CAD build for the part. Positions are in the model's coordinates, mm. A direction names the side the tool comes from. Round coordinates to 2 decimals unless told otherwise and drop trailing zeros. Order: outer loops, then holes, each group sorted by start corner. A loop starts at its lowest first (then second) coordinate and runs counter-clockwise, first axis right, second up. Notation, with made-up numbers: (79, 88.25) - (95, 88.25) arc R27 cw to (95, 119.25) - close; hole circle Ø11 at (-32, -28.5). An arc over 180 degrees is marked (long way). Use one line per item in the form item = value. Start each with the question number.
from build123d import *

# Parameters (mm, degrees)
F0_R     = 9.525
F1_DEPTH = 9.525
F2_DEPTH = 88.9
F3_DEPTH = 25.4


with BuildPart() as f1:
    # F0 (on Front) → F1 (new body)
    with BuildSketch(Plane.XZ):
        Polygon((-4.2214523455, 17.4378681917), (-17.2123630146, 5.0630491238), (-12.9909106691, -12.3748190679), (4.2214523455, -17.4378681917), (17.2123630146, -5.0630491238), (12.9909106691, 12.3748190679), align=None)
        Circle(F0_R, mode=Mode.SUBTRACT)
        Circle(F0_R)
    extrude(amount=F1_DEPTH)

    # F0 (on Front) → F2 (join)
    with BuildSketch(Plane.XZ):
        Circle(F0_R)
    extrude(amount=F2_DEPTH)

    # F3 (add): a face of the model
    f3_faces = [f1.faces().sort_by_distance(p)[0] for p in [
        (0, -88.9, 0),
    ]]
    extrude(f3_faces, amount=F3_DEPTH)


solid = f1.part
(1) Flat gauge pins, fed straight in: P1, Ø4, axis at x = -1, y = -55.5, coming from the -Z side (3 decimals); P2, Ø5, axis at y = -70, z = -9, coming from the -X side; P3, Ø2, axis at y = -33, z = -5, coming from the -X side. Where does each tip first touch, or does it go through?
(2) Slice it at B-B (y = -93.5). Give the cut face in (x, z) (3 decimals), and give its area (3 significant figures).
(3) Wall check: line 1 (Y direction, x = 9.5, z = 2.5) (3 decimals); line 2 (X direction, y = -65, z = -1); line 3 (Z direction, x = 4.5, y = -28). Give the ranges that are in metal, low to high. Write a range as [from, to].
(4) Which spindle directions (+Z, -Z, +X, -X, +Y, -Y) get a long thin tool onto all of the face, cutting with end or side? Do faces 1 (the flat face through (10.626, -4.696, -11.337)), 2 (the cylindrical face through (-7.559, -61.179, -5.796)). Say none if no direction does.
(5) Slice it at C-C (x = 2.5). Give the cut face in (y, z) (1 decimal).
(6) Slice it at A-A (z = 0). Give the cut face in (x, y) (3 decimals), and give its area (3 significant figures).
Results list:
q1.P1 = -9.525
q1.P2 = -6.96
q1.P3 = -8.64
q2.outline = circle Ø19.05 at (0, 0)
q2.area = 285 mm²
q3.line_1 = [-9.525, 0]
q3.line_2 = [-9.47, 9.47]
q3.line_3 = [-8.39, 8.39]
q4.face_1 = -Z, +X, +Y, -Y
q4.face_2 = -Y
q5.outline = (-114.3, -9.2) - (-9.5, -9.2) - (-9.5, -16.9) - (0, -16.9) - (0, 15.5) - (-9.5, 15.5) - (-9.5, 9.2) - (-114.3, 9.2) - close
q6.outline = (-15.987, -9.525) - (-9.525, -9.525) - (-9.525, -114.3) - (9.525, -114.3) - (9.525, -9.525) - (15.987, -9.525) - (15.987, 0) - (-15.987, 0) - close
q6.area = 2,300 mm²
